Design review of the part built by this model. Coordinates are the model's own, in mm. A direction names the side the tool comes from. Give positions to 0.01 mm unless a question says otherwise; leave off trailing zeros. Loops run counter-clockwise (first coordinate to the right, second up) from the corner with the lowest first, then second, coordinate; pieces in that order, holes last.
from build123d import *

# Parameters (mm, degrees)
SKETCH_1_W          = 60
SKETCH_1_H          = 60
EXTRUDE_300_DEPTH   = 22.5
SKETCH_2_W          = 56
SKETCH_2_H          = 56
CUT_EXTRUDE_1_DEPTH = 20.5
SKETCH_4_W          = 10
SKETCH_4_H          = 9
EXTRUDE_2_DEPTH     = 9
SKETCH_5_R          = 1
CUT_EXTRUDE_2_DEPTH = 8.8


with BuildPart() as part:
    # Эскиз1 → Extrude 300 (new body)
    with BuildSketch(Plane.XY):
        Rectangle(SKETCH_1_W, SKETCH_1_H)
    extrude(amount=EXTRUDE_300_DEPTH)

    # Эскиз2 → Вырез-Вытянуть1 (cut)
    with BuildSketch(Plane.XY.offset(22.5)):
        Rectangle(SKETCH_2_W, SKETCH_2_H)
    extrude(amount=-CUT_EXTRUDE_1_DEPTH, mode=Mode.SUBTRACT)

    # Эскиз4 → Бобышка-Вытянуть2 (add)
    with BuildSketch(Plane.XY.offset(2)):
        with Locations((-23, 23.5)):
            Rectangle(SKETCH_4_W, SKETCH_4_H)
    extrude(amount=EXTRUDE_2_DEPTH)

    # Эскиз5 → Вырез-Вытянуть2 (cut)
    with BuildSketch(Plane.XY.offset(11)):
        with Locations((-23, 23.5)):
            Circle(SKETCH_5_R)
    extrude(amount=-CUT_EXTRUDE_2_DEPTH, mode=Mode.SUBTRACT)


solid = part.part
Q1. Tool access review of faces 1 (the face through (-2, -29, 22.5)), 2 (the face through (-23, 24, 2.2)): name each direction out of +Z, -Z, +X, -X, +Y, -Y from which nothing blocks a thin tool from reaching the whole face with its end or side.
Results:
face 1: +Z, +X, -X, +Y, -Y
face 2: +Z
Q2. Insertion check: pin 1 (7 mm diameter, centred on x = -25, y = 23, fed in from +Z); pin 2 (4 mm diameter, centred on x = 4.5, y = 11.5, fed in from +Z). Each pin has a flat end and moves straight along its axis. Give the tip position at first contact, or say it passes through.
Results:
pin 1: stops at z = 22.5
pin 2: stops at z = 2
Q3. Draft analysis for pull direction X (two halves, no side actions). For faces 3 (the face through (30, 0, 11)), 4 (the face through (0, -28, 12)), 5 (the face through (0, 30, 11)), state which applies: pulls with the +X half, pulls with the -X half, needs draft (parallel to the pull), parting line crosses it, or undercut.
Results:
face 3: pulls with the +X half
face 4: undercut
face 5: needs draft
Q4. Take a section at D-D (y = 21.5). Give the boundary of the cut face in (x, z), plus the area to 3 significant figures.
Results:
outline: (-30, 0) - (30, 0) - (30, 22.5) - (28, 22.5) - (28, 2) - (-18, 2) - (-18, 11) - (-28, 11) - (-28, 22.5) - (-30, 22.5) - close
area: 292 mm2
Q5. Take a section at C-C (z = 15.75). Give the boundary of the cut face in (x, y).
Results:
outline: (-30, -30) - (30, -30) - (30, 30) - (-30, 30) - close; hole (-28, -28) - (28, -28) - (28, 28) - (-28, 28) - close
Q6. Take a section at A-A (z = 4.25). Give the boundary of the cut face in (x, y), plus the area to 3 significant figures.
Results:
outline: (-30, -30) - (30, -30) - (30, 30) - (-30, 30) - close; hole (-28, -28) - (28, -28) - (28, 28) - (-18, 28) - (-18, 19) - (-28, 19) - close; hole circle Ø2 at (-23, 23.5)
area: 551 mm2
Q7. Wall thickness on line 1 (Y direction, x = -23, z = 6.5); line 2 (X direction, y = 14, z = 3.75); line 3 (Y direction, x = -27, z = 7): over which ranges is each line inside the solid? List them lowest first.
Results:
line 1: y = -30 to -28, 19 to 22.5, 24.5 to 30
line 2: x = -30 to -28, 28 to 30
line 3: y = -30 to -28, 19 to 30
Q8. Take a section at B-B (x = -12.5). Give the boundary of the cut face in (y, z), plus the area to 3 significant figures.
Results:
outline: (-30, 0) - (30, 0) - (30, 22.5) - (28, 22.5) - (28, 2) - (-28, 2) - (-28, 22.5) - (-30, 22.5) - close
area: 202 mm2
